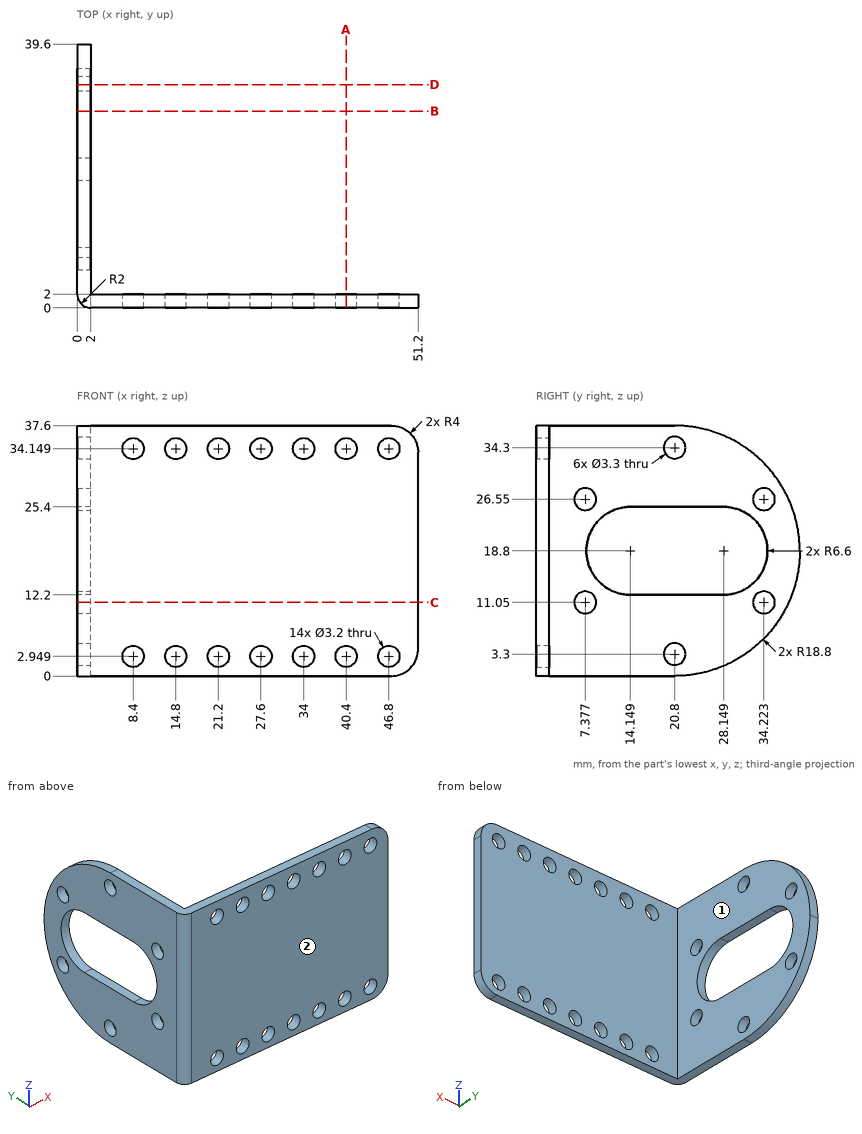
Design review of the part shown in the three views and the two pictorial views. Dimensions are in mm from the part's minimum x, y and z. A direction names the side the tool comes from. Coordinates: 2 decimals unless noted, no trailing zeros. Order: outer loops, then holes, each group sorted by start corner. A loop starts at its lowest first (then second) coordinate and runs counter-clockwise, first axis right, second up.
Item 1: For pin 1 Ø1.9 at (x, z) = (34, 34.15) entering from +Y; pin 2 Ø4 at (x, z) = (40.4, 2.95) entering from +Y; pin 3 Ø4.5 at (y, z) = (7.38, 26.55) entering from +X, all flat-tipped, find the tip position at first contact; note any pin that passes through.
Item 2: Take a section at A-A, the plane x = 40.4. Write out the cut boundary in (y, z).
Item 3: Take a section at C-C, the plane z = 11.05. Write out the cut boundary in (x, y), then the cut area to 3 significant figures.
Item 4: For line 1 (Z direction, x = 21, y = 1) (1 decimal); line 2 (Y direction, x = 1, z = 11) (1 decimal); line 3 (X direction, y = 7, z = 18), list the stretches that pass through material, from the lowest coordinate up.
Item 5: For the marked faces 1 and 2, list the 3-axis set-ups (+Z, -Z, +X, -X, +Y, -Y) from which the entire face can be reached by the end or side of a thin tool; tool diameter is ignored.
Item 6: Take a section at B-B, the plane y = 29.5. Write out the cut boundary in (x, z).
Item 7: Take a section at D-D, the plane y = 33.5. Write out the cut boundary in (x, z).
The answers:
1. pin 1: passes through
1. pin 2: stops at y = 2
1. pin 3: stops at x = 2
2. outline: (0, 0) - (2, 0) - (2, 1.35) - (0, 1.35) - close; (0, 4.55) - (2, 4.55) - (2, 32.55) - (0, 32.55) - close; (0, 35.75) - (2, 35.75) - (2, 37.6) - (0, 37.6) - close
3. outline: (0, 2) arc R2 ccw to (2, 0) - (51.2, 0) - (51.2, 2) - (2, 2) - (2, 5.73) - (0, 5.73) - close; (0, 9.03) - (2, 9.03) - (2, 32.57) - (0, 32.57) - close; (0, 35.87) - (2, 35.87) - (2, 37.93) - (0, 37.93) - close
3. area: 160 mm2
4. line 1: z = 0 to 1.4, 4.5 to 32.6, 35.7 to 37.6
4. line 2: y = 0.3 to 5.7, 9 to 32.6, 35.9 to 37.9
4. line 3: x = 0 to 2
5. face 1: +Z, -Z, +X, +Y
5. face 2: +Z, -Z, +X, -X, -Y
6. outline: (0, 2.13) - (2, 2.13) - (2, 12.34) - (0, 12.34) - close; (0, 25.26) - (2, 25.26) - (2, 35.47) - (0, 35.47) - close
7. outline: (0, 4.94) - (2, 4.94) - (2, 9.57) - (0, 9.57) - close; (0, 12.53) - (2, 12.53) - (2, 14.94) - (0, 14.94) - close; (0, 22.66) - (2, 22.66) - (2, 25.07) - (0, 25.07) - close; (0, 28.03) - (2, 28.03) - (2, 32.66) - (0, 32.66) - close
